from build123d import *

# Parameters (mm, degrees)
SKETCH1_W           = 42.3
SKETCH1_H           = 42.3
BOSS_EXTRUDE1_DEPTH = 34
CHAMFER2_SIZE       = 2
SKETCH2_R           = 11
BOSS_EXTRUDE2_DEPTH = 2
SKETCH3_R           = 2.5
CUT_EXTRUDE2_DEPTH  = 20
SKETCH5_W           = 15
SKETCH5_H           = 9.5
BOSS_EXTRUDE4_DEPTH = 5


with BuildPart() as part:
    # Sketch1 → Boss-Extrude1 (new body)
    with BuildSketch(Plane(origin=(0, 0, 0), x_dir=(1, 0, 0), z_dir=(0, 1, 0))):
        with Locations((21.15, 21.15)):
            Rectangle(SKETCH1_W, SKETCH1_H)
    extrude(amount=BOSS_EXTRUDE1_DEPTH)

    # Chamfer2
    chamfer2_edges = [part.edges().sort_by_distance(p)[0] for p in [
        (0, 17, -42.3),
        (42.3, 17, -42.3),
        (42.3, 17, 0),
        (0, 17, 0),
    ]]
    chamfer(chamfer2_edges, length=CHAMFER2_SIZE)

    # Sketch2 → Boss-Extrude2 (add)
    with BuildSketch(Plane(origin=(0, 34, 0), x_dir=(1, 0, 0), z_dir=(0, 1, 0))):
        with Locations(Location((21.15, 21.15, 0), (0, 0, 270))):
            Circle(SKETCH2_R)
    extrude(amount=BOSS_EXTRUDE2_DEPTH)

    # Sketch3 → Cut-Extrude2 (cut)
    with BuildSketch(Plane(origin=(0, 36, 0), x_dir=(1, 0, 0), z_dir=(0, 1, 0))):
        with Locations(Location((21.15, 21.15, 0), (0, 0, 270))):
            Circle(SKETCH3_R)
    extrude(amount=-CUT_EXTRUDE2_DEPTH, mode=Mode.SUBTRACT)

    # Sketch5 → Boss-Extrude4 (add)
    with BuildSketch(Plane.XY):
        with Locations((21.15, 4.75)):
            Rectangle(SKETCH5_W, SKETCH5_H)
    extrude(amount=BOSS_EXTRUDE4_DEPTH)


solid = part.part
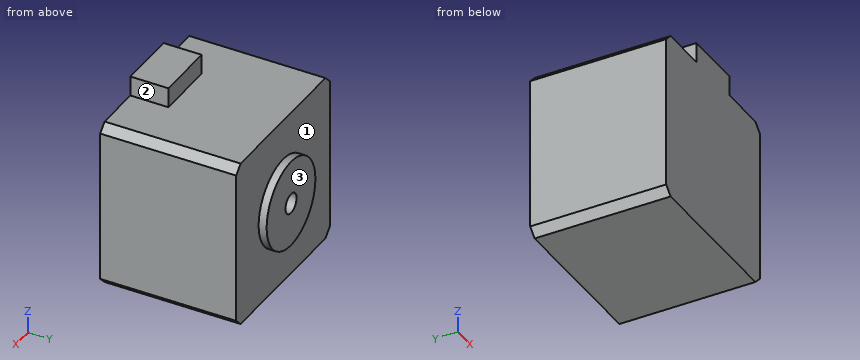
The model under review builds one solid part; all positions refer to its coordinate system, in mm. Face numbers are marked on the shaded views. A direction names the side the tool comes from. Coordinates: 2 decimals unless noted, no trailing zeros. Write each loop counter-clockwise with the first axis right and the second up, starting at its lowest first coordinate (ties: lowest second). Pieces come first, ordered by that corner, then holes. Notation, with made-up numbers: (-19.75, 20) - (14.25, 20) arc R27 cw to (14.25, 43) - close; hole circle Ø1 at (48, 81.5). An arc over 180 degrees is marked (long way). Answer as a JSON object with one key per item and string values. Group by question number.
1. Clearance check with flat-ended pins moving along their axes: pin 1 Ø17 at (x, y) = (26, 17) entering from +Z; pin 2 Ø4 at (x, z) = (32, -5) entering from +Y; pin 3 Ø5.5 at (y, z) = (2.5, 1.5) entering from +X; pin 4 Ø1.5 at (y, z) = (6.5, 2) entering from -X. State where each tip first meets the part, or that it passes through.
2. Add section C-C (z = -21.15). Give the boundary of the cut face in (x, y), plus the area to 3 significant figures.
3. Add section B-B (x = 21.15). Give the boundary of the cut face in (y, z).
4. To check wall thickness, follow probe 1 along Z at (x, y) = (21, 26); probe 2 along X at (y, z) = (22.5, -21.15); probe 3 along Y at (x, z) = (28, -30). State the ranges of each line that lie inside material, in increasing order.
5. Machinability: for the marked faces 1, 2 and 3, which of the approach directions +Z, -Z, +X, -X, +Y, -Y give a long, thin tool a straight path to every point of the face, cutting with its end or side? Answer none if there is none.
6. Add section A-A (y = 22). Give the boundary of the cut face in (x, z), plus the area to 3 significant figures.
7. Add section D-D (y = 4). Give the boundary of the cut face in (x, z), plus the area to 3 significant figures.
Findings:
{
 "1": {"pin 1": "z = 5", "pin 2": "y = 34", "pin 3": "x = 41.55", "pin 4": "x = 13.65"},
 "2": {"outline": "(0, 0) - (42.3, 0) - (42.3, 34) - (32.15, 34) - (32.15, 36) - (23.65, 36) - (23.65, 16) - (18.65, 16) - (18.65, 36) - (10.15, 36) - (10.15, 34) - (0, 34) - close", "area": "1,380 mm²"},
 "3": {"outline": "(0, -42.3) - (34, -42.3) - (34, -32.15) - (36, -32.15) - (36, -23.65) - (16, -23.65) - (16, -18.65) - (36, -18.65) - (36, -10.15) - (34, -10.15) - (34, 0) - (9.5, 0) - (9.5, 5) - (0, 5) - close"},
 "4": {"probe 1": "-42.3 to -23.65, -18.65 to 0", "probe 2": "0 to 18.65, 23.65 to 42.3", "probe 3": "0 to 34"},
 "5": {"face 1": "+Y", "face 2": "+Z, +X, +Y, -Y", "face 3": "+Z, -Z, +X, -X, +Y"},
 "6": {"outline": "(0, -40.3) - (2, -42.3) - (40.3, -42.3) - (42.3, -40.3) - (42.3, -2) - (40.3, 0) - (2, 0) - (0, -2) - close; hole circle Ø5 at (21.15, -21.15)", "area": "1,760 mm²"},
 "7": {"outline": "(0, -40.3) - (2, -42.3) - (40.3, -42.3) - (42.3, -40.3) - (42.3, -2) - (40.3, 0) - (28.65, 0) - (28.65, 5) - (13.65, 5) - (13.65, 0) - (2, 0) - (0, -2) - close", "area": "1,860 mm²"}
}
